Answer from the drawing. Dimensions are ordinates in mm from the lowest x, y and z of the part. A direction names the side the tool comes from. Give positions to 0.01 mm unless a question says otherwise; leave off trailing zeros. Write each loop counter-clockwise with the first axis right and the second up, starting at its lowest first coordinate (ties: lowest second). Pieces come first, ordered by that corner, then holes. Notation, with made-up numbers: (-33, -3.75) -> (26, -3.75) arc R29 cw to (26, 29.25) -> close; hole circle Ø10 at (38.25, 83.25). An arc over 180 degrees is marked (long way). Write item = value, one per line.
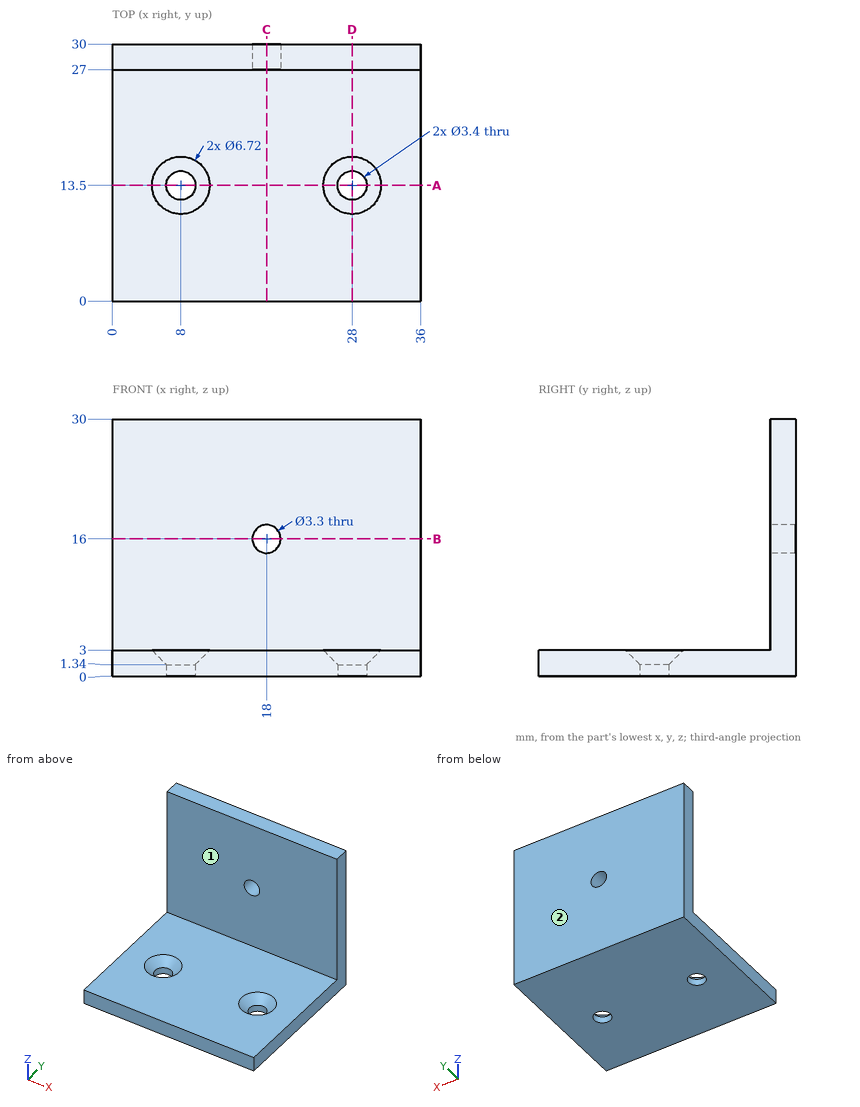
(1) A tool of negligible diameter and unlimited length cuts with its end or side. For the marked faces 1 and 2, from which of +Z, -Z, +X, -X, +Y, -Y can it reach the whole face along a straight path? Write none if from no direction.
Checks:
face_1 = +Z, +X, -X, -Y
face_2 = +Z, -Z, +X, -X, +Y
(2) Given P1, Ø2, axis at x = 10, z = 22.5, coming from the -Y side; P2, Ø5, axis at x = 16.5, y = 8.5, coming from the +Z side; P3, Ø2.5, axis at x = 8, y = 13.5, coming from the +Z side, each flat-ended and moving along its own axis, determine where each tip first touches the part or whether it passes through.
Checks:
P1 = 27
P2 = 3
P3 = through
(3) Consider L1, parallel to X at y = 13.5, z = 1; L2, parallel to Z at x = 18, y = 29.35; L3, parallel to X at y = 29.4, z = 16. Determine where each line is inside the solid, lowest interval first.
Checks:
L1 = 0 to 6.3, 9.7 to 26.3, 29.7 to 36
L2 = 0 to 14.35, 17.65 to 30
L3 = 0 to 16.35, 19.65 to 36
(4) The part is cut by section B-B on z = 16. Determine the outline of the cut face in (x, y).
Checks:
outline = (0, 27) -> (16.35, 27) -> (16.35, 30) -> (0, 30) -> close; (19.65, 27) -> (36, 27) -> (36, 30) -> (19.65, 30) -> close
(5) The part is cut by section D-D on x = 28. Determine the outline of the cut face in (y, z).
Checks:
outline = (0, 0) -> (11.8, 0) -> (11.8, 1.34) -> (10.14, 3) -> (0, 3) -> close; (15.2, 0) -> (30, 0) -> (30, 30) -> (27, 30) -> (27, 3) -> (16.86, 3) -> (15.2, 1.34) -> close
(6) The part is cut by section C-C on x = 18. Determine the outline of the cut face in (y, z).
Checks:
outline = (0, 0) -> (30, 0) -> (30, 14.35) -> (27, 14.35) -> (27, 3) -> (0, 3) -> close; (27, 17.65) -> (30, 17.65) -> (30, 30) -> (27, 30) -> close
(7) The part is cut by section A-A on y = 13.5. Determine the outline of the cut face in (x, z), plus the area to 3 significant figures.
Checks:
outline = (0, 0) -> (6.3, 0) -> (6.3, 1.34) -> (4.64, 3) -> (0, 3) -> close; (9.7, 0) -> (26.3, 0) -> (26.3, 1.34) -> (24.64, 3) -> (11.36, 3) -> (9.7, 1.34) -> close; (29.7, 0) -> (36, 0) -> (36, 3) -> (31.36, 3) -> (29.7, 1.34) -> close
area = 82.1 mm²
